Here's how the part is built. I have some questions about the finished solid (model axes, mm). A direction names the side the tool comes from. Coordinates: 2 decimals unless noted, no trailing zeros. Order: outer loops, then holes, each group sorted by start corner. A loop starts at its lowest first (then second) coordinate and runs counter-clockwise, first axis right, second up. Notation, with made-up numbers: (-36, 9.25) -> (-28, 9.25) arc R12 ccw to (-28, 19.25) -> close; hole circle Ø9 at (13.5, 49). An arc over 180 degrees is marked (long way). One line per item, written item: value. Start each with the question number.
```python
from build123d import *

# Parameters (mm, degrees)
F0_W         = 38.1
F0_H         = 66.675
F1_DEPTH     = 3.175
F2_T1_DEPTH  = 57.15
F2_T3_DEPTH  = 101.6
F2_T6_ANGLE  = 90
F2_T8_ANGLE  = 90
F2_T10_ANGLE = 90
F2_T12_ANGLE = 90


# Not quite as in the source:
# - a fillet or chamfer that OpenCascade refuses, or shapes differently, is made with other operations: its cross-section is extruded or revolved along the edge and cut away or added


with BuildPart() as f1:
    # F0 (on Front) → F1 (new body)
    with BuildSketch(Plane.XZ):
        with BuildLine():
            ThreePointArc((0, 6.35), (1.8598719395, 1.8598719395), (6.35, 0))
            Line((6.35, 0), (63.5, 0))
            ThreePointArc((63.5, 0), (67.9901280605, 1.8598719395), (69.85, 6.35))
            Line((69.85, 6.35), (69.85, 107.95))
            ThreePointArc((69.85, 107.95), (67.9901280605, 112.4401280605), (63.5, 114.3))
            Line((63.5, 114.3), (6.35, 114.3))
            ThreePointArc((6.35, 114.3), (1.8598719395, 112.4401280605), (0, 107.95))
            Line((0, 107.95), (0, 6.35))
        make_face()
        with Locations((34.925, 57.15)):
            Rectangle(F0_W, F0_H, mode=Mode.SUBTRACT)
    extrude(amount=F1_DEPTH)

    # F2: fillet of radius 5.08 on 1 edges, made by hand

    # F2_s2 → F2_t1 (cut)
    with BuildSketch(Plane.YZ.offset(6.35)):
        with BuildLine():
            ThreePointArc((0, 114.3), (-2.3071134838, 112.4305202921), (-3.175, 109.5907139607))
            Line((-3.175, 109.5907139607), (-3.175, 114.3))
            Line((-3.175, 114.3), (0, 114.3))
        make_face()
        with BuildLine():
            ThreePointArc((0, 0), (-2.3071134838, 1.8694797079), (-3.175, 4.7092860393))
            Line((-3.175, 4.7092860393), (-3.175, 0))
            Line((-3.175, 0), (0, 0))
        make_face()
    extrude(amount=F2_T1_DEPTH, mode=Mode.SUBTRACT)

    # F2_s4 → F2_t3 (cut)
    with BuildSketch(Plane.XY.offset(6.35)):
        with BuildLine():
            ThreePointArc((0, 0), (1.8694797079, -2.3071134838), (4.7092860393, -3.175))
            Line((4.7092860393, -3.175), (0, -3.175))
            Line((0, -3.175), (0, 0))
        make_face()
        with BuildLine():
            ThreePointArc((69.85, 0), (67.9805202921, -2.3071134838), (65.1407139607, -3.175))
            Line((65.1407139607, -3.175), (69.85, -3.175))
            Line((69.85, -3.175), (69.85, 0))
        make_face()
    extrude(amount=F2_T3_DEPTH, mode=Mode.SUBTRACT)

    # F2_s5 → F2_t6 (revolve, cut)
    with BuildSketch(Plane.XY.offset(107.95)):
        with BuildLine():
            ThreePointArc((69.85, 0), (67.9805202921, -2.3071134838), (65.1407139607, -3.175))
            Line((65.1407139607, -3.175), (69.85, -3.175))
            Line((69.85, -3.175), (69.85, 0))
        make_face()
    revolve(axis=Axis((63.5, -3.175, 107.95), (0, -1, 0)), revolution_arc=F2_T6_ANGLE, mode=Mode.SUBTRACT)

    # F2_s7 → F2_t8 (revolve, cut)
    with BuildSketch(Plane.YZ.offset(6.35)):
        with BuildLine():
            ThreePointArc((0, 114.3), (-2.3071134838, 112.4305202921), (-3.175, 109.5907139607))
            Line((-3.175, 109.5907139607), (-3.175, 114.3))
            Line((-3.175, 114.3), (0, 114.3))
        make_face()
    revolve(axis=Axis((6.35, -3.175, 107.95), (0, -1, 0)), revolution_arc=F2_T8_ANGLE, mode=Mode.SUBTRACT)

    # F2_s9 → F2_t10 (revolve, cut)
    with BuildSketch(Plane.XY.offset(6.35)):
        with BuildLine():
            ThreePointArc((0, 0), (1.8694797079, -2.3071134838), (4.7092860393, -3.175))
            Line((4.7092860393, -3.175), (0, -3.175))
            Line((0, -3.175), (0, 0))
        make_face()
    revolve(axis=Axis((6.35, -3.175, 6.35), (0, -1, 0)), revolution_arc=F2_T10_ANGLE, mode=Mode.SUBTRACT)

    # F2_s11 → F2_t12 (revolve, cut)
    with BuildSketch(Plane.YZ.offset(63.5)):
        with BuildLine():
            ThreePointArc((0, 0), (-2.3071134838, 1.8694797079), (-3.175, 4.7092860393))
            Line((-3.175, 4.7092860393), (-3.175, 0))
            Line((-3.175, 0), (0, 0))
        make_face()
    revolve(axis=Axis((63.5, -3.175, 6.35), (0, -1, 0)), revolution_arc=F2_T12_ANGLE, mode=Mode.SUBTRACT)


solid = f1.part
```
Q1. Imagine slicing it at A-A (x = 40). Write out the boundary of the cut face in (y, z) (1 decimal), plus the area to 3 significant figures.
Q2. I need wall thicknesses on line 1 (Z direction, x = 21.5, y = -0.45); line 2 (X direction, y = -0.85, z = 35) (3 decimals); line 3 (Z direction, x = 20.5, y = -0.75). Which ranges of each line are inside material? Lowest first, please.
Q3. Imagine slicing it at C-C (z = 99.5). Write out the boundary of the cut face in (x, y) (3 decimals), plus the area to 3 significant figures.
Q4. If we mould it in two halves opening along Z, with no side actions, what happens to faces 1 (the face through (34.52, -2.28, 112.47)), 2 (the face through (53.975, -2, 57)), 3 (the face through (1.83, -2.28, 56.44))? For each: +Z half, -Z half, draft (parallel to the pull), parting line (faces both ways), or undercut.
Q5. Imagine slicing it at B-B (z = 75). Write out the boundary of the cut face in (x, y) (3 decimals).
Q6. For P1, Ø1, axis at x = 40, y = -1.5, coming from the -Z side; P2, Ø1.5, axis at x = 17.5, y = -1.5, coming from the -Z side; P3, Ø1.5, axis at x = 53, z = 27, coming from the +Y side; P4, Ø1.6, axis at y = -1, z = 47, coming from the +X side, each with a flat end and sliding along its axis, tell me the tip position at first contact or that it passes through.
Q7. Imagine slicing it at D-D (x = 62). Write out the boundary of the cut face in (y, z) (3 decimals).
Q8. For faces 4 (the face through (34.52, -2.28, 1.83)), 5 (the face through (15.875, -2, 57)), which set-ups out of +Z, -Z, +X, -X, +Y, -Y let a thin tool reach every point of the face, with its end or its side?
Completed:
1. outline: (-3.2, 4.7) arc R5.1 ccw to (0, 0) -> (0, 23.8) -> (-3.2, 23.8) -> close; (-3.2, 90.5) -> (0, 90.5) -> (0, 114.3) arc R5.1 ccw to (-3.2, 109.6) -> close
1. area: 143 mm2
2. line 1: z = 0.21 to 23.81, 90.49 to 114.09
2. line 2: x = 0.441 to 15.875, 53.975 to 69.409
2. line 3: z = 0.38 to 23.81, 90.49 to 113.92
3. outline: (0, 0) arc R5.08 ccw to (4.709, -3.175) -> (65.141, -3.175) arc R5.08 ccw to (69.85, 0) -> close
3. area: 214 mm2
4. face 1: +Z half
4. face 2: undercut
4. face 3: draft
5. outline: (0, 0) arc R5.08 ccw to (4.709, -3.175) -> (15.875, -3.175) -> (15.875, 0) -> close; (53.975, -3.175) -> (65.141, -3.175) arc R5.08 ccw to (69.85, 0) -> (53.975, 0) -> close
6. P1: stops at z = 0.54
6. P2: stops at z = 0.38
6. P3: passes through
6. P4: stops at x = 69.76
7. outline: (-3.175, 4.709) arc R5.08 ccw to (0, 0) -> (0, 114.3) arc R5.08 ccw to (-3.175, 109.591) -> close
8. face 4: -Z, +X, -X, -Y
8. face 5: +Y, -Y
